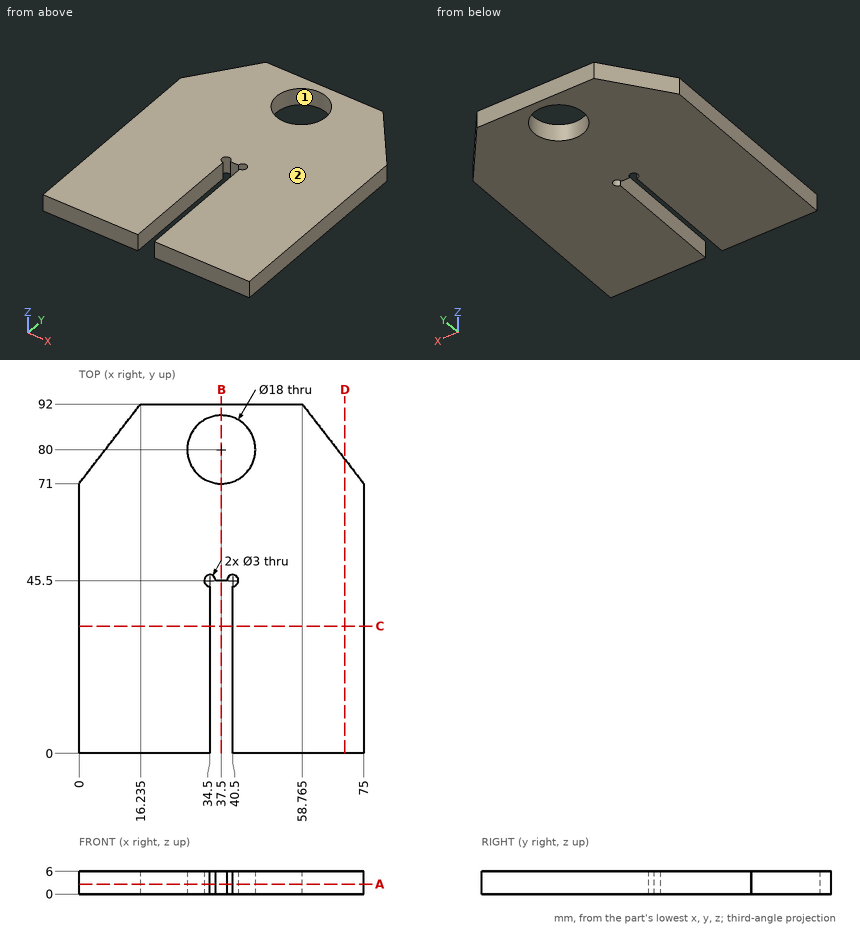
Could you check a few things on this drawing? It's one solid part, dimensions in mm from its lowest x, y, z. Coordinates: 2 decimals unless noted, no trailing zeros. Write each loop counter-clockwise with the first axis right and the second up, starting at its lowest first coordinate (ties: lowest second). Pieces come first, ordered by that corner, then holes. Notation, with made-up numbers: M 76.5,36.5 L 117.5,36.5 A17 ccw 117.5,47.5 Z; hole C 88.25,46.5 d3. An arc over 180 degrees is marked long. Answer as CSV lines item,"result". Start each with the question number.
Q1. Suppose I cut it at B-B, the plane x = 37.5. List the corners of the cut face in (y, z) for me.
Q2. Will these pins go through, and if not, where does the flat tip stop? pin 1 Ø11 at (x, y) = (37.5, 80) entering from +Z; pin 2 Ø1.5 at (x, z) = (37.5, 4.5) entering from -Y.
Q3. Suppose I cut it at D-D, the plane x = 70. List the corners of the cut face in (y, z) for me.
Q4. Suppose I cut it at C-C, the plane y = 33.5. List the corners of the cut face in (x, z) for me.
Q5. Suppose I cut it at A-A, the plane z = 2.6. List the corners of the cut face in (x, y) for me (1 decimal), then the cut area to 3 significant figures.
Q6. If we mould it in two halves opening along X, with no side actions, what happens to the marked faces 1 and 2? For each: pulls with the +X half, pulls with the -X half, needs draft (parallel to the pull), parting line crosses it, or undercut.
Q7. I need wall thicknesses on probe 1 along Y at (x, z) = (38, 3.75); probe 2 along X at (y, z) = (20.5, 0.7); probe 3 along Y at (x, z) = (45, 1.7) (1 decimal). Which ranges of each line are inside material? Lowest first, please. Write a range as [from, to].
Entries:
1,outline,"M 45.5,0 L 71,0 L 71,6 L 45.5,6 Z; M 89,0 L 92,0 L 92,6 L 89,6 Z"
2,pin 1,"passes through"
2,pin 2,"stops at y = 45.5"
3,outline,"M 0,0 L 77.47,0 L 77.47,6 L 0,6 Z"
4,outline,"M 0,0 L 34.5,0 L 34.5,6 L 0,6 Z; M 40.5,0 L 75,0 L 75,6 L 40.5,6 Z"
5,outline,"M 0,0 L 34.5,0 L 34.5,44 A1.5 cw long 36,45.5 L 39,45.5 A1.5 cw long 40.5,44 L 40.5,0 L 75,0 L 75,71 L 58.8,92 L 16.2,92 L 0,71 Z; hole C 37.5,80 d18"
5,area,"6,020 mm²"
6,face 1,"undercut"
6,face 2,"needs draft"
7,probe 1,"y = [45.5, 71.01], [88.99, 92]"
7,probe 2,"x = [0, 34.5], [40.5, 75]"
7,probe 3,"y = [0, 75], [85, 92]"
